Here's how the part is built. I have some questions about the finished solid (model axes, mm). A direction names the side the tool comes from. Give positions to 0.01 mm unless a question says otherwise; leave off trailing zeros. Loops run counter-clockwise (first coordinate to the right, second up) from the corner with the lowest first, then second, coordinate; pieces in that order, holes last. Notation, with made-up numbers: M 24.5,29.25 L 66.5,29.25 A21 ccw 66.5,58.25 Z; hole C 58.5,10 d6. An arc over 180 degrees is marked long. Answer as CSV lines item,"result". Start each with the question number.
Item 1: For faces 5 (the cylindrical face through (-15.641, 0.203, -14.085)), 6 (the cylindrical face through (-3.21, 0.2, -11.44)), which set-ups out of +Z, -Z, +X, -X, +Y, -Y let a thin tool reach every point of the face, with its end or its side?
Item 2: I want a section at A-A on x = -8.9. List the corners of the cut face in (y, z) for me.
Item 3: I want a section at C-C on z = 14.76. List the corners of the cut face in (x, y) for me.
Item 4: Will this pin go through, and if not, where does the flat tip stop? P1, Ø1.8, axis at x = -14.76, z = -14.76, coming from the -Y side.
Item 5: If we mould it in two halves opening along X, with no side actions, what happens to faces 1 (the cylindrical face through (-3.24, 0.2, 11.39)), 2 (the cylindrical face through (-12.1, 0.2, 8)), 3 (the cylindrical face through (-12.1, 0.2, -7.9)), 4 (the flat face through (-10, 0, 0))? For each: released by +X, released by -X, zero draft, split by the parting line, or undercut.
Item 6: If I drill on line 1 along Z through (x, y) = (-13, 0.1); line 2 along Z through (x, y) = (-8.9, 0.2); line 3 along Z through (x, y) = (-14.5, 0.1), over which ranges is the centre line in solid material (lowest first)? Write a range as from..to.
Item 7: I want a section at B-B on y = 0.3. List the corners of the cut face in (x, z) for me, plus the area to 3 significant figures.
Item 8: I want a section at D-D on x = -14.76. List the corners of the cut face in (y, z) for me, plus the area to 3 significant figures.
Autodesk Inventor part; units mm, degrees
ref_plane "YZ Plane" through (0, 0, 0) normal (1, 0, 0) x (0, 1, 0)
ref_plane "XZ Plane" through (0, 0, 0) normal (0, 1, 0) x (-1, 0, 0)
ref_plane "XY Plane" through (0, 0, 0) normal (0, 0, 1) x (1, 0, 0)
sketch "Sketch1" plane through (0, 0, 0) normal (0, 1, 0) x (-1, 0, 0)
  line L0 (16, 16) -> (-16, 16)
  line L1 (-16, 16) -> (-16, -16)
  line L2 (-16, -16) -> (16, -16)
  line L3 (16, -16) -> (16, 16)
  line L4 (16, 16) -> (-16, -16) construction
  line L5 (-16, 16) -> (16, -16) construction
  point P0 (0, 0)
  dimension "d0" = 32
  dimension "d1" = 32
extrude "Extrusion1" add sketch "Sketch1" along normal blind 0.4
sketch "Sketch2" plane through (0, 0.4, 0) normal (0, 1, 0) x (1, 0, 0)
  line L0 (-9.5, -9.5) -> (9.5, -9.5)
  line L1 (9.5, -9.5) -> (9.5, 9.5)
  line L2 (9.5, 9.5) -> (-9.5, 9.5)
  line L3 (-9.5, 9.5) -> (-9.5, -9.5)
  line L4 (-9.5, -9.5) -> (9.5, 9.5) construction
  line L5 (9.5, -9.5) -> (-9.5, 9.5) construction
  circle A0 centre (0, 9.5) radius 3.75
  circle A1 centre (0, -9.5) radius 3.75
  point P0 (0, 0)
  point P1 (-3.75, -9.5)
  point P2 (3.75, -9.5)
  point P3 (3.75, 9.5)
  point P4 (-3.75, 9.5)
  dimension "d4" = 19
  dimension "d5" = 19
  dimension "d6" = 7.5
  dimension "d7" = 7.5
extrude "Extrusion2" cut sketch "Sketch2" against normal blind 0.4
sketch "Sketch3" plane through (0, 0.4, 0) normal (0, 1, 0) x (1, 0, 0)
  line L0 (-16, -16) -> (16, -16)
  line L1 (16, 16) -> (-16, 16)
  line L2 (0, -16) -> (16, -16)
  line L3 (16, -16) -> (16, 16)
  line L4 (16, 16) -> (0, 16)
  line L5 (0, 16) -> (0, -16)
  point P0 (0, 0)
extrude "Extrusion3" cut sketch "Sketch3" against normal blind 0.4
sketch "Sketch4" plane through (0, 0.4, 0) normal (0, 1, 0) x (1, 0, 0)
  circle A0 centre (-14.76, -14.76) radius 1.11
  circle A1 centre (-14.76, 14.76) radius 1.11
  line L0 (-16, 16) -> (-16, -16)
  line L1 (-16, -16) -> (0, -16)
  line L2 (0, 16) -> (-16, 16)
  circle A2 centre (0, -14.4) radius 2.4
  circle A3 centre (-14.5, 7.96) radius 2.4
  circle A4 centre (-14.5, -7.96) radius 2.4
  circle A5 centre (-8.9, -14.2) radius 2.4
  circle A6 centre (-8.9, 14.2) radius 2.4
  circle A7 centre (0, 14.4) radius 2.4
  line L3 (0, -16) -> (0, -13.25)
  line L4 (0, 13.25) -> (0, 16)
  point P0 (0, 0)
  point P1 (-7.3125, -16)
  point P2 (-10.4875, -16)
  point P3 (-10.4875, 16)
  point P4 (-7.3125, 16)
  point P5 (-16, -6.0865)
  point P6 (-16, -9.8335)
  point P7 (-16, 9.8335)
  point P8 (-16, 6.0865)
  dimension "d12" = 2.22
  dimension "d13" = 2.22
  dimension "d14" = 1.24
  dimension "d15" = 1.24
  dimension "d16" = 1.24
  dimension "d17" = 1.24
  dimension "d18" = 4.8
  dimension "d19" = 4.8
  dimension "d20" = 4.8
  dimension "d21" = 4.8
  dimension "d22" = 4.8
  dimension "d23" = 4.8
  dimension "d24" = 0
  dimension "d26" = 0
  dimension "d28" = 7.1
  dimension "d29" = 1.8
  dimension "d30" = 1.8
  dimension "d31" = 7.1
  dimension "d32" = 1.6
  dimension "d33" = 1.6
  dimension "d34" = 1.5
  dimension "d35" = 8.04
  dimension "d36" = 8.04
  dimension "d37" = 1.5
extrude "Extrusion4" cut sketch "Sketch4" against normal blind 0.4 contours A0 | A1 | A2 | A5 L1 | A4 L0 | A3 L0 | A7 | L2 A6 picked at (-8.777, -14.4925) picked at (-14.5551, -7.8666) picked at (-14.7976, 7.5771) picked at (-8.6453, 14.6416)
properties part number "Top Cover Power Side"
Result:
1,face 5,"+Y, -Y"
1,face 6,"+X, +Y, -Y"
2,outline,"M 0,-11.8 L 0.4,-11.8 L 0.4,-9.5 L 0,-9.5 Z; M 0,9.5 L 0.4,9.5 L 0.4,11.8 L 0,11.8 Z"
3,outline,"M -16,0 L -15.87,0 L -15.87,0.4 L -16,0.4 Z; M -13.65,0 L -11.23,0 L -11.23,0.4 L -13.65,0.4 Z; M -6.57,0 L -2.37,0 L -2.37,0.4 L -6.57,0.4 Z"
4,P1,"through"
5,face 1,"released by +X"
5,face 2,"undercut"
5,face 3,"undercut"
5,face 4,"zero draft"
6,line 1,"-16..-9.83, -6.09..6.09, 9.83..16"
6,line 2,"-11.8..-9.5, 9.5..11.8"
6,line 3,"-16..-15.84, -13.68..-10.36, -5.56..5.56, 10.36..13.68, 15.84..16"
7,outline,"M -16,-16 L -10.49,-16 A2.4 cw long -7.31,-16 L -1.79,-16 A2.4 cw -1.79,-12.8 A3.75 cw -3.75,-9.5 L -9.5,-9.5 L -9.5,9.5 L -3.75,9.5 A3.75 cw -1.79,12.8 A2.4 cw -1.79,16 L -7.31,16 A2.4 cw long -10.49,16 L -16,16 L -16,9.83 A2.4 cw long -16,6.09 L -16,-6.09 A2.4 cw long -16,-9.83 Z; hole C -14.76,-14.76 d2.22; hole C -14.76,14.76 d2.22"
7,area,"224 mm^2"
8,outline,"M 0,-16 L 0.4,-16 L 0.4,-15.87 L 0,-15.87 Z; M 0,-13.65 L 0.4,-13.65 L 0.4,-10.35 L 0,-10.35 Z; M 0,-5.57 L 0.4,-5.57 L 0.4,5.57 L 0,5.57 Z; M 0,10.35 L 0.4,10.35 L 0.4,13.65 L 0,13.65 Z; M 0,15.87 L 0.4,15.87 L 0.4,16 L 0,16 Z"
8,area,"7.21 mm^2"
